The listing builds one solid part. Answer for the finished solid, in the listing's coordinates (mm). Face numbers are marked on the shaded views. A direction names the side the tool comes from. Round coordinates to 2 decimals unless told otherwise and drop trailing zeros. Write each loop counter-clockwise with the first axis right and the second up, starting at its lowest first coordinate (ties: lowest second). Pieces come first, ordered by that corner, then holes.
(1) A cutting plane is placed at B-B, the plane z = 0. Give the vertices of the cut face in (x, y).
(2) Find the intervals of material crossed by probe 1 along X at (y, z) = (0.15, 0); probe 2 along X at (y, z) = (-0.2, 0); probe 3 along Y at (x, z) = (2.4, 0.3), in increasing order.
(3) A cutting plane is placed at C-C, the plane y = -0.2. Give the vertices of the cut face in (x, z), and give its area (3 significant figures).
(4) The mould has two halves that part along Y. Classify the marked faces 3, 4 and 5: +Y half, -Y half, draft (parallel to the pull), parting line (faces both ways), or undercut.
(5) For the marked faces 1 and 2, determine the directions among +Z, -Z, +X, -X, +Y, -Y from which every point of the face is accessible in a straight line to the end or side of a thin tool.
(6) A cutting plane is placed at D-D, the plane x = -1.35. Give the vertices of the cut face in (y, z), and give its area (3 significant figures).
(7) A cutting plane is placed at A-A, the plane x = 0. Give the vertices of the cut face in (y, z), and give its area (3 significant figures).
from build123d import *

# Parameters (mm, degrees)
SKETCH1_R           = 2.1
BOSS_EXTRUDE1_DEPTH = 1
SKETCH2_R           = 2.95
BOSS_EXTRUDE2_DEPTH = 0.5
SKETCH3_R           = 0.2
CUT_EXTRUDE1_DEPTH  = 5.43339599


with BuildPart() as part:
    # Sketch1 → Boss-Extrude1 (new body)
    with BuildSketch(Plane(origin=(0, 0, 0), x_dir=(1, 0, 0), z_dir=(0, 1, 0))):
        with Locations(Location((0, 0, 0), (0, 0, 270))):
            Circle(SKETCH1_R)
    extrude(amount=BOSS_EXTRUDE1_DEPTH)

    # Sketch2 → Boss-Extrude2 (add)
    with BuildSketch(Plane.XZ):
        with Locations(Location((0, 0, 0), (0, 0, 270))):
            Circle(SKETCH2_R)
    extrude(amount=BOSS_EXTRUDE2_DEPTH)

    # Sketch3 → Cut-Extrude1 (cut, through all)
    with BuildSketch(Plane(origin=(0, 1, 0), x_dir=(1, 0, 0), z_dir=(0, 1, 0))):
        with Locations(Location((0, 0, 0), (0, 0, 270))):
            Circle(SKETCH3_R)
    extrude(amount=-CUT_EXTRUDE1_DEPTH, mode=Mode.SUBTRACT)


solid = part.part
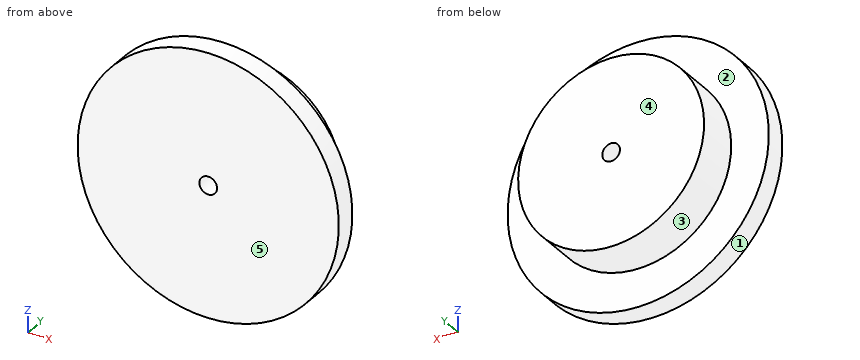
Solutions:
1. outline: (-2.95, -0.5) - (-0.2, -0.5) - (-0.2, 1) - (-2.1, 1) - (-2.1, 0) - (-2.95, 0) - close; (0.2, -0.5) - (2.95, -0.5) - (2.95, 0) - (2.1, 0) - (2.1, 1) - (0.2, 1) - close
2. probe 1: x = -2.1 to -0.2, 0.2 to 2.1
2. probe 2: x = -2.95 to -0.2, 0.2 to 2.95
2. probe 3: y = -0.5 to 0
3. outline: circle Ø5.9 at (0, 0); hole circle Ø0.4 at (0, 0)
3. area: 27.2 mm2
4. face 3: draft
4. face 4: +Y half
4. face 5: -Y half
5. face 1: +Y, -Y
5. face 2: +Y
6. outline: (-0.5, -2.62) - (0, -2.62) - (0, -1.61) - (1, -1.61) - (1, 1.61) - (0, 1.61) - (0, 2.62) - (-0.5, 2.62) - close
6. area: 5.84 mm2
7. outline: (-0.5, -2.95) - (0, -2.95) - (0, -2.1) - (1, -2.1) - (1, -0.2) - (-0.5, -0.2) - close; (-0.5, 0.2) - (1, 0.2) - (1, 2.1) - (0, 2.1) - (0, 2.95) - (-0.5, 2.95) - close
7. area: 6.55 mm2
